Check sheet for the modelled part. Datum: model origin and axes. Units: mm. A direction names the side the tool comes from. Give positions to 0.01 mm unless a question says otherwise; leave off trailing zeros. Order: outer loops, then holes, each group sorted by start corner. A loop starts at its lowest first (then second) coordinate and runs counter-clockwise, first axis right, second up.
Autodesk Inventor part; units mm, degrees
ref_plane "YZ Plane" through (0, 0, 0) normal (1, 0, 0) x (0, 1, 0)
ref_plane "XZ Plane" through (0, 0, 0) normal (0, 1, 0) x (-1, 0, 0)
ref_plane "XY Plane" through (0, 0, 0) normal (0, 0, 1) x (1, 0, 0)
sketch "Sketch1" plane through (0, 0, 0) normal (0, 0, 1) x (1, 0, 0)
  line L0 (0, 0) -> (15, 0)
  line L1 (15, 0) -> (15, 4)
  line L2 (15, 4) -> (0, 4)
  line L3 (0, 4) -> (0, 0)
  line L4 (0, 53.5) -> (15, 53.5)
  line L5 (15, 53.5) -> (15, 49.5)
  line L6 (15, 49.5) -> (0, 49.5)
  line L7 (0, 49.5) -> (0, 53.5)
  line L8 (0, 53.5) -> (-7.7, 53.5)
  line L9 (-7.7, 53.5) -> (-7.7, -10.5)
  line L10 (-7.7, -10.5) -> (0, -10.5)
  line L11 (0, -10.5) -> (0, 53.5)
  point P0 (0, 49.5)
  dimension "d0" = 15
  dimension "d1" = 4
  dimension "d2" = 15
  dimension "d3" = 4
  dimension "d4" = 45.5
  dimension "d5" = 7.7
  dimension "d6" = 64
extrude "Extrusion1" add sketch "Sketch1" along normal mid plane 45
extrude "Extrusion2" cut sketch "Sketch1" along normal mid plane 30 contours L3 L2 L1 L0
sketch "Sketch3" plane through (0, 49.5, 22.5) normal (0, -1, 0) x (1, 0, 0)
  line L0 (0, 0) -> (15, 0)
  line L1 (7.5, 0) -> (7.5, -45)
  line L2 (15, -45) -> (0, -45)
  circle A0 centre (7.5, -3.75) radius 1.55
  circle A1 centre (7.5, -7.5) radius 1.55
  circle A2 centre (7.5, -22.5) radius 1.55
  circle A3 centre (7.5, -37.5) radius 1.55
  circle A4 centre (7.5, -41.25) radius 1.55
  line L3 (0, 0) -> (15, 0)
  line L4 (15, -45) -> (0, -45)
  line L5 (15, -45) -> (15, 0)
  point P0 (0, -22.5)
  dimension "d11" = 3.1
  dimension "d12" = 3.1
  dimension "d13" = 3.1
  dimension "d14" = 3.1
  dimension "d15" = 3.1
  dimension "d16" = 3.75
  dimension "d17" = 7.5
  dimension "d18" = 3.75
  dimension "d19" = 7.5
  dimension "d20" = 7.5
extrude "Extrusion3" cut sketch "Sketch3" along normal through all contours A0 L1 | L1 A0 | A4 L1 | L1 A4
extrude "Extrusion4" cut sketch "Sketch3" against normal through all contours A1 L1 | L1 A1 | A2 L1 | L1 A2 | A3 L1 | L1 A3
sketch "Sketch4" plane through (0, 4, -22.5) normal (1, 0, 0) x (0, 0, -1)
  circle A0 centre (-22.5, -1.5) radius 6
  line L0 (-45, -14.5) -> (0, -14.5)
  line L1 (-22.5, -1.5) -> (-22.5, -14.5) construction
  point P0 (-22.5, -4)
  dimension "d29" = 12
  dimension "d40" = 13
extrude "Extrusion6" cut sketch "Sketch4" against normal through all
fillet "Fillet1" radius 2 14 edges at (0, 49.5, 0) (15, 49.5, 0) (15, 53.5, 0) (-7.7, 53.5, 0) (0, 4, 18.75) (0, 4, -18.75) (15, 4, -18.75) (15, 0, -18.75) (15, 4, 18.75) (15, 0, 18.75) (0, -10.5, 0) (0, 0, 18.75) (0, 0, -18.75) (-7.7, -10.5, 0)
properties part number "ThickBearingBracket" material "PC/ABS Plastic"
1) Material ranges on L1, parallel to Z at x = 7.5, y = 51.25; L2, parallel to Y at x = -3.75, z = 0; L3, parallel to Z at x = 3.75, y = 3.5, recorded low to high.
Recorded:
L1: z = -22.5 to -16.55, -13.45 to -1.55, 1.55 to 13.45, 16.55 to 22.5
L2: y = -10.5 to -3.5, 8.5 to 53.5
L3: z = -22.5 to -15, 15 to 22.5
2) Set-up check for faces 4 (the face through (7.298, 2.028, -20.287)), 5 (the face through (7, 0, 17)), 6 (the face through (8, 4, 17)), 7 (the face through (7, 2, 15)): record each of +Z, -Z, +X, -X, +Y, -Y from which the full face is reachable in a straight line by a thin tool's end or side.
Recorded:
face 4: -Y
face 5: +Z, -Z, +X, -Y
face 6: +Z, -Z, +X
face 7: +X, -Y
3) Section check B-B, the plane x = 7.5. State how many separate pieces and enclosed holes the cut face has, then the cut area to 3 significant figures.
Recorded:
separate pieces: 8
enclosed holes: 0
area: 178 mm2
4) Section check A-A, the plane y = 1. Record the cut outline in (x, z).
Recorded:
outline: (-7.7, -22.5) - (14.73, -22.5) - (14.73, -15) - (0, -15) - (0, -5.81) - (-7.7, -5.81) - close; (-7.7, 5.81) - (0, 5.81) - (0, 15) - (14.73, 15) - (14.73, 22.5) - (-7.7, 22.5) - close; hole circle Ø3.1 at (7.5, -18.75); hole circle Ø3.1 at (7.5, 18.75)
5) Draft check along Z on faces 1 (the face through (7.298, 2.028, 17.213)), 2 (the face through (-2, 22, -22.5)), 3 (the face through (0.57, -0.6, -18.8)). Enter one of: +Z half, -Z half, draft (parallel to the pull), parting line (faces both ways), or undercut.
Recorded:
face 1: undercut
face 2: -Z half
face 3: draft
6) Depth check by flat-ended pin: pin 1 Ø2.5 at (x, z) = (7.5, -18.75) entering from -Y; pin 2 Ø4 at (x, z) = (7, -19.5) entering from -Y; pin 3 Ø10 at (y, z) = (42, -15) entering from +X. Enter the tip coordinate at first touch or a pass-through.
Recorded:
pin 1: stops at y = 49.5
pin 2: stops at y = 0
pin 3: stops at x = 0
